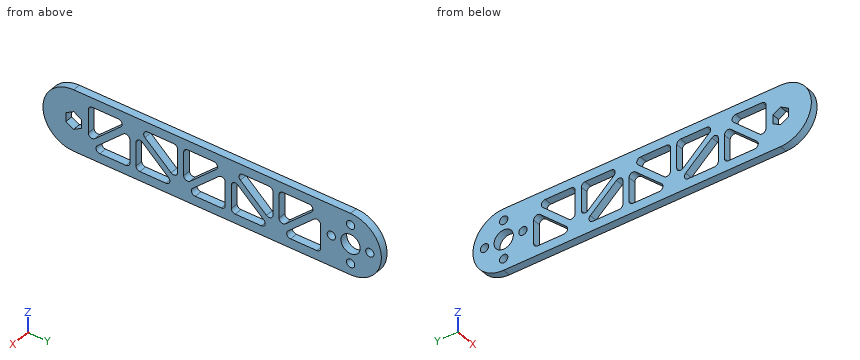
from build123d import *

# Parameters (mm, degrees)
SKETCH1_R           = 7.9375
SKETCH1_R_2         = 3.429
BOSS_EXTRUDE1_DEPTH = 6.35
CUT_EXTRUDE2_DEPTH  = 7.35
FILLET2_R           = 3.175


with BuildPart() as part:
    # Sketch1 → Boss-Extrude1 (new body)
    with BuildSketch(Plane(origin=(0, 0, 0), x_dir=(0, 0, -1), z_dir=(1, 0, 0))):
        with BuildLine():
            Line((-25.4, 228.6), (-25.4, 0))
            ThreePointArc((-25.4, 0), (0, -25.4), (25.4, 0))
            Line((25.4, 0), (25.4, 228.6))
            ThreePointArc((25.4, 228.6), (0, 254), (-25.4, 228.6))
        make_face()
        with Locations((0, 228.6)):
            Circle(SKETCH1_R, mode=Mode.SUBTRACT)
        with Locations((0, 212.725)):
            Circle(SKETCH1_R_2, mode=Mode.SUBTRACT)
        with Locations((-15.875, 228.6)):
            Circle(SKETCH1_R_2, mode=Mode.SUBTRACT)
        with Locations((0, 244.475)):
            Circle(SKETCH1_R_2, mode=Mode.SUBTRACT)
        with Locations((15.875, 228.6)):
            Circle(SKETCH1_R_2, mode=Mode.SUBTRACT)
        Polygon((7.332348419, 0), (3.666174209, 6.35), (-3.666174209, 6.35), (-7.332348419, 0), (-3.666174209, -6.35), (3.666174209, -6.35), align=None, mode=Mode.SUBTRACT)
    extrude(amount=BOSS_EXTRUDE1_DEPTH)

    # Sketch3 → Cut-Extrude2 (cut, through all)
    with BuildSketch(Plane(origin=(6.35, 0, 0), x_dir=(0, 0, -1), z_dir=(1, 0, 0))):
        Polygon((-12.06309933, 203.835), (17.78, 170.794425741), (17.78, 203.835), align=None)
        Polygon((-17.78, 202.585574259), (-17.78, 169.545), (12.06309933, 169.545), align=None)
        Polygon((12.063099331, 164.465), (-17.78, 164.465), (-17.78, 131.424425736), align=None)
        Polygon((17.78, 163.215574258), (-12.063099331, 130.174999995), (17.78, 130.174999995), align=None)
        Polygon((12.063099331, 90.804999989), (-17.78, 123.845574253), (-17.78, 90.804999989), align=None)
        Polygon((17.78, 125.094999995), (-12.063099331, 125.094999995), (17.78, 92.054425731), align=None)
        Polygon((17.78, 51.434999984), (17.78, 84.475574248), (-12.063099331, 51.434999984), align=None)
        Polygon((12.063099331, 85.724999989), (-17.78, 85.724999989), (-17.78, 52.684425726), align=None)
        Polygon((17.78, 46.354999984), (-12.063099329, 46.354999984), (17.78, 13.31442574), align=None)
        Polygon((12.063099329, 12.065), (-17.78, 45.105574244), (-17.78, 12.065), align=None)
    extrude(amount=-CUT_EXTRUDE2_DEPTH, mode=Mode.SUBTRACT)

    # Fillet2
    fillet2_edges = [part.edges().sort_by_distance(p)[0] for p in [
        (3.175, 52.684425726, 17.78),
        (3.175, 85.724999989, 17.78),
        (3.175, 46.354999984, 12.063099329),
        (3.175, 46.354999984, -17.78),
        (3.175, 13.31442574, -17.78),
        (3.175, 169.545, -12.06309933),
        (3.175, 169.545, 17.78),
        (3.175, 202.585574259, 17.78),
        (3.175, 164.465, -12.063099331),
        (3.175, 131.424425736, 17.78),
        (3.175, 164.465, 17.78),
        (3.175, 130.174999995, 12.063099331),
        (3.175, 163.215574258, -17.78),
        (3.175, 130.174999995, -17.78),
        (3.175, 90.804999989, -12.063099331),
        (3.175, 90.804999989, 17.78),
        (3.175, 123.845574253, 17.78),
        (3.175, 12.065, 17.78),
        (3.175, 45.105574244, 17.78),
        (3.175, 12.065, -12.063099329),
        (3.175, 203.835, 12.06309933),
        (3.175, 203.835, -17.78),
        (3.175, 170.794425741, -17.78),
        (3.175, 125.094999995, 12.063099331),
        (3.175, 125.094999995, -17.78),
        (3.175, 92.054425731, -17.78),
        (3.175, 51.434999984, 12.063099331),
        (3.175, 84.475574248, -17.78),
        (3.175, 51.434999984, -17.78),
        (3.175, 85.724999989, -12.063099331),
    ]]
    fillet(fillet2_edges, radius=FILLET2_R)


solid = part.part
Geometry: final body of the model. Coordinates: model frame, mm. Coordinates: 2 decimals unless noted, no trailing zeros. Loops run counter-clockwise (first coordinate to the right, second up) from the corner with the lowest first, then second, coordinate; pieces in that order, holes last. Notation, with made-up numbers: M -37,-22 L -15,-22 A15 ccw -15,-12 Z; hole C -18,15.25 d7. An arc over 180 degrees is marked long. One line per item, written item: value. Start each with the question number.
1) Pin query (flat end, axial travel): P1, Ø3, axis at x = 1.5, z = 0, coming from the -Y side; P2, Ø2, axis at x = 1.5, z = -7, coming from the -Y side; P3, Ø3, axis at x = 3.5, z = -5, coming from the +Y side. Return the tip coordinate at first contact, or that it passes through.
2) Cut plane A-A (y = 25.5). Return loops of the section in (x, z).
3) Material intervals for L1, parallel to Z at x = 4.5, y = 70; L2, parallel to Z at x = 5, y = 41; L3, parallel to Z at x = 0.5, y = 178, sorted ascending. Write a range as from..to.
4) Cut plane B-B (z = 0). Count the separate pieces of the cut face and the enclosed holes in it, then the cut area to 3 significant figures.
Evaluation:
1. P1: y = -25.4
1. P2: y = -24.68
1. P3: y = 253.76
2. outline: M 0,-25.4 L 6.35,-25.4 L 6.35,-17.78 L 0,-17.78 Z; M 0,-6.77 L 6.35,-6.77 L 6.35,0.07 L 0,0.07 Z; M 0,17.78 L 6.35,17.78 L 6.35,25.4 L 0,25.4 Z
3. L1: -25.4..-17.78, -4.71..2.14, 17.78..25.4
3. L2: -25.4..-17.78, 7.23..25.4
3. L3: -25.4..-17.6, -11.27..-4.43, 17.78..25.4
4. separate pieces: 15
4. enclosed holes: 0
4. area: 658 mm^2
